Could you check a few things on this model? Use its own coordinates, in mm. Face numbers are marked on the shaded views. A direction names the side the tool comes from. Give positions to 0.01 mm unless a question says otherwise; leave off trailing zeros. Loops run counter-clockwise (first coordinate to the right, second up) from the corner with the lowest first, then second, coordinate; pieces in that order, holes last. Notation, with made-up numbers: M 47.5,-25.75 L 55.5,-25.75 A25 cw 55.5,8.25 Z; hole C -40,22 d7. An arc over 180 degrees is marked long. Return JSON: item names as keys, results as strings. Group by question number.
1. Please list where these lines run through material, in increasing order: line 1 (X direction, y = 38.5, z = -6); line 2 (Y direction, x = 79.5, z = -7.5); line 3 (Y direction, x = 184, z = -21).
2. For the marked faces 1 and 2, which set-ups out of +Z, -Z, +X, -X, +Y, -Y let a thin tool reach every point of the face, with its end or its side?
3. If we section it at C-C (x = 262): Write out the boundary of the cut face in (y, z), plus the area to 3 significant figures.
4. If we section it at B-B (y = 44): Write out the boundary of the cut face in (x, z), plus the area to 3 significant figures.
5. If we mould it in two halves opening along X, with no side actions, what happens to the marked faces 3 and 4? For each: +X half, -X half, draft (parallel to the pull), parting line (faces both ways), or undercut.
6. For pin 1 (1.5 mm diameter, centred on y = 43, z = 4, fed in from +X); pin 2 (18 mm diameter, centred on x = 32.5, z = -12, fed in from +Y); pin 3 (13.5 mm diameter, centred on y = 34.5, z = -8, fed in from -X); pin 4 (17.5 mm diameter, centred on y = 26.15, z = -8.85, fed in from -X), each with a flat end and sliding along its axis, tell me the tip position at first contact or that it passes through.
7. If we section it at A-A (z = -8.85): Write out the boundary of the cut face in (x, y).
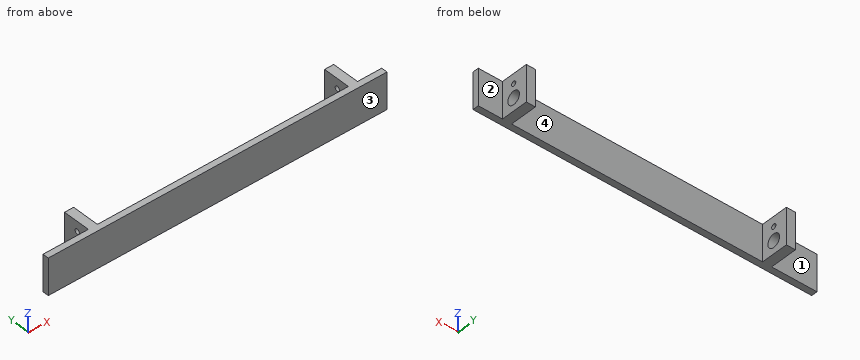
```python
from build123d import *

# Parameters (mm, degrees)
SKETCH2_W           = 60
SKETCH2_H           = 10
BOSS_EXTRUDE1_DEPTH = 560
SKETCH4_W           = 15
SKETCH4_H           = 60
BOSS_EXTRUDE2_DEPTH = 45
SKETCH5_W           = 15
SKETCH5_H           = 60
BOSS_EXTRUDE3_DEPTH = 45
SKETCH6_R           = 11
SKETCH6_R_2         = 4
CUT_EXTRUDE1_DEPTH  = 455


with BuildPart() as part:
    # Sketch2 → Boss-Extrude1 (new body)
    with BuildSketch(Plane(origin=(0, 0, 0), x_dir=(0, 0, -1), z_dir=(1, 0, 0))):
        Rectangle(SKETCH2_W, SKETCH2_H)
    extrude(amount=BOSS_EXTRUDE1_DEPTH)

    # Sketch4 → Boss-Extrude2 (add)
    with BuildSketch(Plane(origin=(0, 5, 0), x_dir=(1, 0, 0), z_dir=(0, 1, 0))):
        with Locations((82.5, 0)):
            Rectangle(SKETCH4_W, SKETCH4_H)
    extrude(amount=BOSS_EXTRUDE2_DEPTH)

    # Sketch5 → Boss-Extrude3 (add)
    with BuildSketch(Plane(origin=(0, 5, 0), x_dir=(1, 0, 0), z_dir=(0, 1, 0))):
        with Locations((512.5, 0)):
            Rectangle(SKETCH5_W, SKETCH5_H)
    extrude(amount=BOSS_EXTRUDE3_DEPTH)

    # Sketch6 → Cut-Extrude1 (cut)
    with BuildSketch(Plane.ZY.offset(-75)):
        with Locations((-8.85, 26.15)):
            Circle(SKETCH6_R)
        with Locations((13.717950956, 26.15)):
            Circle(SKETCH6_R_2)
    extrude(amount=-CUT_EXTRUDE1_DEPTH, mode=Mode.SUBTRACT)


solid = part.part
```
Answer:
{
 "1": {"line 1": "x = 75 to 90, 505 to 520", "line 2": "y = -5 to 15.23, 37.07 to 50", "line 3": "y = -5 to 5"},
 "2": {"face 1": "+Z, -Z, -X, +Y", "face 2": "+Z, -Z, +X, +Y"},
 "3": {"outline": "M -5,-30 L 5,-30 L 5,30 L -5,30 Z", "area": "600 mm²"},
 "4": {"outline": "M 75,-30 L 90,-30 L 90,30 L 75,30 Z; M 505,-30 L 520,-30 L 520,30 L 505,30 Z", "area": "1,800 mm²"},
 "5": {"face 3": "draft", "face 4": "undercut"},
 "6": {"pin 1": "stops at x = 520", "pin 2": "stops at y = 5", "pin 3": "stops at x = 75", "pin 4": "passes through"},
 "7": {"outline": "M 0,-5 L 560,-5 L 560,5 L 520,5 L 520,15.15 L 505,15.15 L 505,5 L 90,5 L 90,15.15 L 75,15.15 L 75,5 L 0,5 Z; M 75,37.15 L 90,37.15 L 90,50 L 75,50 Z; M 505,37.15 L 520,37.15 L 520,50 L 505,50 Z"}
}
